Check sheet for the modelled part. Datum: model origin and axes. Units: mm. A direction names the side the tool comes from. Round coordinates to 2 decimals unless told otherwise and drop trailing zeros. Loops run counter-clockwise (first coordinate to the right, second up) from the corner with the lowest first, then second, coordinate; pieces in that order, holes last. Notation, with made-up numbers: (54, 79) - (84, 79) arc R33 cw to (84, 115) - close; hole circle Ø3 at (50.5, 11.5). An arc over 180 degrees is marked (long way). Return JSON: item names as keys, results as strings.
from build123d import *

# Parameters (mm, degrees)
SKETCH1_W             = 100
SKETCH1_H             = 213.5
BOSS_EXTRUDE1_DEPTH   = 3
BOSS_EXTRUDE1_2_DEPTH = 3
SKETCH2_W             = 300
SKETCH2_H             = 80
BOSS_EXTRUDE2_DEPTH   = 3
SKETCH4_W             = 3
SKETCH4_H             = 213.5
BOSS_EXTRUDE4_DEPTH   = 30
SKETCH5_W             = 94
SKETCH5_H             = 213.5
BOSS_EXTRUDE5_DEPTH   = 3
CUT_EXTRUDE2_REACH    = 195.272
CUT_EXTRUDE1_REACH    = 204.349
SKETCH3_W             = 95
SKETCH3_H             = 10
SKETCH7_W             = 213.5
SKETCH7_H             = 77
BOSS_EXTRUDE6_DEPTH   = 3
SKETCH8_R             = 1.75
CUT_EXTRUDE3_DEPTH    = 277.783760362
CUT_EXTRUDE4_REACH    = 330.594
FILLET1_R             = 5


with BuildPart() as part:
    # Sketch1 → Boss-Extrude1 (new body)
    with BuildSketch(Plane(origin=(0, 0, 0), x_dir=(1, 0, 0), z_dir=(0, 1, 0))):
        with Locations((-100, 0)):
            Rectangle(SKETCH1_W, SKETCH1_H)
    extrude(amount=BOSS_EXTRUDE1_DEPTH)



with BuildPart() as body_2:
    # Sketch1 → Boss-Extrude1 2 (new body)
    with BuildSketch(Plane(origin=(0, 0, 0), x_dir=(1, 0, 0), z_dir=(0, 1, 0))):
        with Locations((100, 0)):
            Rectangle(SKETCH1_W, SKETCH1_H)
    extrude(amount=BOSS_EXTRUDE1_2_DEPTH)


with BuildPart() as part_1:
    add(part.part)

    add(body_2.part)  # Boss-Extrude2 merges body 2
    # Sketch2 → Boss-Extrude2 (add)
    with BuildSketch(Plane.XY.offset(106.75)):
        with Locations((0, -37)):
            Rectangle(SKETCH2_W, SKETCH2_H)
    boss_extrude2 = extrude(amount=BOSS_EXTRUDE2_DEPTH)

    # Mirror1: Boss-Extrude2 across plane
    add(boss_extrude2.mirror(Plane.XY))

    # Sketch4 → Boss-Extrude4 (add)
    with BuildSketch(Plane(origin=(0, 3, 0), x_dir=(1, 0, 0), z_dir=(0, 1, 0))):
        with Locations((-48.5, 0)):
            Rectangle(SKETCH4_W, SKETCH4_H)
        with Locations((48.5, 0)):
            Rectangle(SKETCH4_W, SKETCH4_H)
    extrude(amount=-BOSS_EXTRUDE4_DEPTH)

    # Sketch5 → Boss-Extrude5 (add)
    with BuildSketch(Plane.XZ.offset(27)):
        Rectangle(SKETCH5_W, SKETCH5_H)
    extrude(amount=-BOSS_EXTRUDE5_DEPTH)

    # Sketch6 → Cut-Extrude2 (cut, up to next)
    with BuildSketch(Plane(origin=(0, -24, 0), x_dir=(1, 0, 0), z_dir=(0, 1, 0)), mode=Mode.PRIVATE) as cut_extrude2_sk1:
        Polygon((-35.5, 106.75), (35.5, 106.75), (35.5, 101.75), (4.5, 101.75), (4.5, 96.75), (-4.5, 96.75), (-4.5, 101.75), (-35.5, 101.75), align=None)
    cut_extrude2_tool1 = extrude(cut_extrude2_sk1.sketch, amount=-CUT_EXTRUDE2_REACH, mode=Mode.PRIVATE) & part_1.part
    # Sketch6 → Cut-Extrude2 (cut, up to next)
    with BuildSketch(Plane(origin=(0, -24, 0), x_dir=(1, 0, 0), z_dir=(0, 1, 0)), mode=Mode.PRIVATE) as cut_extrude2_sk2:
        Polygon((-35.5, -106.75), (35.5, -106.75), (35.5, -101.75), (4.5, -101.75), (4.5, -96.75), (-4.5, -96.75), (-4.5, -101.75), (-35.5, -101.75), align=None)
    cut_extrude2_tool2 = extrude(cut_extrude2_sk2.sketch, amount=-CUT_EXTRUDE2_REACH, mode=Mode.PRIVATE) & part_1.part
    add(cut_extrude2_tool1.solids().sort_by_distance((0, -24, -103.6875))[0], mode=Mode.SUBTRACT)
    add(cut_extrude2_tool2.solids().sort_by_distance((0, -24, 103.6875))[0], mode=Mode.SUBTRACT)

    # Sketch3 → Cut-Extrude1 (cut, up to next)
    with BuildSketch(Plane(origin=(0, 3, 0), x_dir=(1, 0, 0), z_dir=(0, 1, 0)), mode=Mode.PRIVATE) as cut_extrude1_sk1:
        with Locations((-87.5, 0)):
            Rectangle(SKETCH3_W, SKETCH3_H)
    cut_extrude1_tool1 = extrude(cut_extrude1_sk1.sketch, amount=-CUT_EXTRUDE1_REACH, mode=Mode.PRIVATE) & part_1.part
    # Sketch3 → Cut-Extrude1 (cut, up to next)
    with BuildSketch(Plane(origin=(0, 3, 0), x_dir=(1, 0, 0), z_dir=(0, 1, 0)), mode=Mode.PRIVATE) as cut_extrude1_sk2:
        with Locations((87.5, 0)):
            Rectangle(SKETCH3_W, SKETCH3_H)
    cut_extrude1_tool2 = extrude(cut_extrude1_sk2.sketch, amount=-CUT_EXTRUDE1_REACH, mode=Mode.PRIVATE) & part_1.part
    add(cut_extrude1_tool1.solids().sort_by_distance((-87.5, 3, 0))[0], mode=Mode.SUBTRACT)
    add(cut_extrude1_tool2.solids().sort_by_distance((87.5, 3, 0))[0], mode=Mode.SUBTRACT)

    # Sketch7 → Boss-Extrude6 (add)
    with BuildSketch(Plane.ZY.offset(150)):
        with Locations((0, -38.5)):
            Rectangle(SKETCH7_W, SKETCH7_H)
    boss_extrude6 = extrude(amount=-BOSS_EXTRUDE6_DEPTH)

    # Mirror2: Boss-Extrude6 across plane
    add(boss_extrude6.mirror(Plane(origin=(0, 0, 0), x_dir=(0, 0, 1), z_dir=(1, 0, 0))))

    # Sketch8 → Cut-Extrude3 (cut, through all)
    with BuildSketch(Plane.XY.offset(109.75)):
        with Locations((-25, -13)):
            Circle(SKETCH8_R)
        with Locations((25, -13)):
            Circle(SKETCH8_R)
        with BuildLine():
            Line((-14, -63), (-14, -77))
            Line((-14, -77), (-6, -77))
            Line((-6, -77), (-6, -63))
            ThreePointArc((-6, -63), (-10, -59), (-14, -63))
        make_face()
        with BuildLine():
            Line((14, -63), (14, -77))
            Line((14, -77), (6, -77))
            Line((6, -77), (6, -63))
            ThreePointArc((6, -63), (10, -59), (14, -63))
        make_face()
    extrude(amount=-CUT_EXTRUDE3_DEPTH, mode=Mode.SUBTRACT)

    # Sketch10 → Cut-Extrude4 (cut, up to next)
    with BuildSketch(Plane(origin=(150, 0, 0), x_dir=(0, 0, -1), z_dir=(1, 0, 0)), mode=Mode.PRIVATE) as cut_extrude4_sk1:
        with BuildLine():
            Line((-30, -27), (30, -27))
            ThreePointArc((30, -27), (33.535533906, -28.464466094), (35, -32))
            Line((35, -32), (35, -77))
            Line((35, -77), (-35, -77))
            Line((-35, -77), (-35, -32))
            ThreePointArc((-35, -32), (-33.535533906, -28.464466094), (-30, -27))
        make_face()
    cut_extrude4_tool1 = extrude(cut_extrude4_sk1.sketch, amount=-CUT_EXTRUDE4_REACH, mode=Mode.PRIVATE) & part_1.part
    add(cut_extrude4_tool1.solids().sort_by_distance((150, -52.073445, 0))[0], mode=Mode.SUBTRACT)

    # Fillet1
    fillet1_edges = [part_1.edges().sort_by_distance(p)[0] for p in [
        (148.5, -77, 35),
        (148.5, -77, -35),
    ]]
    fillet(fillet1_edges, radius=FILLET1_R)


solid = part_1.part
Q1. Scan lines: probe 1 along X at (y, z) = (-25, -76.5); probe 2 along Z at (x, y) = (-95.5, -61); probe 3 along Y at (x, z) = (25, -107). Record each from-to range of solid material in increasing order. Write a range as [from, to].
Answer key:
{"probe 1": "x = [-150, -147], [-50, 50], [147, 150]", "probe 2": "z = [-109.75, -106.75], [106.75, 109.75]", "probe 3": "y = [-77, -14.75], [-11.25, 3]"}
Q2. Sectioned sample at D-D (z = 83). Enter the section's corners in (x, y), plus the area to 3 significant figures.
Answer key:
{"outline": "(-150, -77) - (-147, -77) - (-147, 0) - (-50, 0) - (-50, -27) - (50, -27) - (50, 0) - (147, 0) - (147, -77) - (150, -77) - (150, 3) - (47, 3) - (47, -24) - (-47, -24) - (-47, 3) - (-150, 3) - close", "area": "1,520 mm²"}
Q3. Tool access check on faces 4 (the face through (47, -10, -55)), 5 (the face through (50, -13, -55)), 6 (the face through (-80.7, 0.3, 5)). Record the directions out of +Z, -Z, +X, -X, +Y, -Y that give a thin tool (end or side, any length) a straight path to the whole face; none if there is none.
Answer key:
{"face 4": "+Y", "face 5": "-Y", "face 6": "+Y, -Y"}
Q4. Depth check by flat-ended pin: P1, Ø1.5, axis at x = 10.5, z = 75, coming from the +Y side; P2, Ø3, axis at x = -67.5, z = -40.5, coming from the -Y side; P3, Ø0.9, axis at x = 148.5, z = 12.5, coming from the -Y side. Enter the tip coordinate at first touch or a pass-through.
Answer key:
{"P1": "stops at y = -24", "P2": "stops at y = 0", "P3": "stops at y = -27"}
Q5. Sectioned sample at B-B (x = -123.5). Enter the section's corners in (y, z).
Answer key:
{"outline": "(-77, -109.75) - (3, -109.75) - (3, -5) - (0, -5) - (0, -106.75) - (-77, -106.75) - close; (-77, 106.75) - (0, 106.75) - (0, 5) - (3, 5) - (3, 109.75) - (-77, 109.75) - close"}
Q6. Draft check along Z on faces 1 (the face through (-99, 0, 22)), 2 (the face through (113, -77, -109)), 3 (the face through (-2, -36, -109.75)). Enter one of: released by +Z, released by -Z, zero draft, split by the parting line, or undercut.
Answer key:
{"face 1": "undercut", "face 2": "zero draft", "face 3": "released by -Z"}
Q7. Sectioned sample at A-A (x = -0.5). Enter the section's corners in (y, z), plus the area to 3 significant figures.
Answer key:
{"outline": "(-77, -109.75) - (3, -109.75) - (3, -106.75) - (-77, -106.75) - close; (-77, 106.75) - (3, 106.75) - (3, 109.75) - (-77, 109.75) - close; (-27, -96.75) - (-24, -96.75) - (-24, 96.75) - (-27, 96.75) - close", "area": "1,060 mm²"}
Q8. Sectioned sample at C-C (y = -47). Enter the section's corners in (x, z).
Answer key:
{"outline": "(-150, -109.75) - (150, -109.75) - (150, -35) - (147, -35) - (147, -106.75) - (-147, -106.75) - (-147, 106.75) - (147, 106.75) - (147, 35) - (150, 35) - (150, 109.75) - (-150, 109.75) - close"}
